Input: part model. Units: mm. Frame: model coordinates. Face numbers are marked on the shaded views. A direction names the side the tool comes from. Give positions to 0.01 mm unless a question says otherwise; leave off trailing zeros. Order: outer loops, then holes, each group sorted by start corner. A loop starts at its lowest first (then second) coordinate and runs counter-clockwise, first axis right, second up. Notation, with made-up numbers: (13, -4) - (17, -4) arc R28 ccw to (17, 18) - close; hole circle Ø10 at (88.25, -2.5). An arc over 180 degrees is marked (long way). Answer in a Markdown table with one row per item. Add a question column.
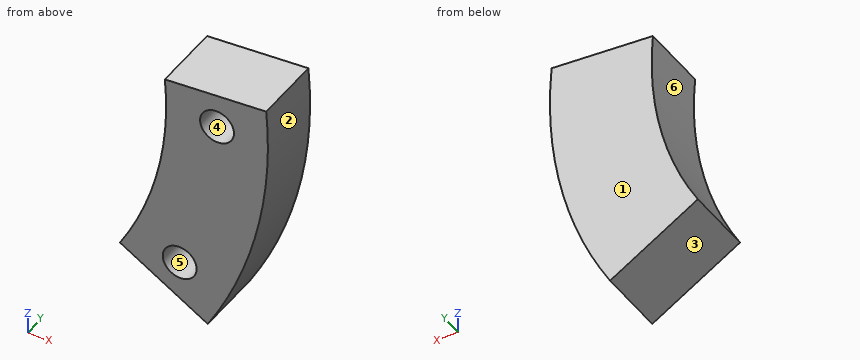
from build123d import *

# Parameters (mm, degrees)
BOSS_EXTRUDE1_DEPTH       = 10
F_5_0MM_DOWEL_HOLE1_D     = 5
F_5_0MM_DOWEL_HOLE1_DEPTH = 6
F_5_0MM_DOWEL_HOLE1_TIP   = 1.502151548


with BuildPart() as part:
    # Sketch1 → Boss-Extrude1 (new body)
    with BuildSketch(Plane(origin=(0, 0, 0), x_dir=(1, 0, 0), z_dir=(0, 1, 0))):
        with BuildLine():
            ThreePointArc((49.589984709, -4.345321229), (48.569954781, 10.909073863), (42.968659609, 25.134492066))
            Line((42.968659609, 25.134492066), (55.916226787, 32.708163842))
            ThreePointArc((55.916226787, 32.708163842), (63.205336897, 14.196259639), (64.532728193, -5.654678771))
            Line((64.532728193, -5.654678771), (49.589984709, -4.345321229))
        make_face()
    extrude(amount=BOSS_EXTRUDE1_DEPTH)

    # Ø5.0mm Dowel Hole1
    with Locations(Plane(origin=(0, 0, 0), x_dir=(-1, 0, 0), z_dir=(0, -1, 0))):
        with Locations((-57.28, 0), (-51.776228177, 24.499399905)):
            Hole(F_5_0MM_DOWEL_HOLE1_D / 2, depth=F_5_0MM_DOWEL_HOLE1_DEPTH)
            with Locations((0, 0, -(F_5_0MM_DOWEL_HOLE1_DEPTH + F_5_0MM_DOWEL_HOLE1_TIP / 2))):  # 118° drill point
                Cone(0, F_5_0MM_DOWEL_HOLE1_D / 2, F_5_0MM_DOWEL_HOLE1_TIP, mode=Mode.SUBTRACT)


solid = part.part
Q1. Section B-B, the plane z = -21. Return loops of the section in (x, y).
Q2. Section A-A, the plane y = 7. Return loops of the section in (x, z), then the cut area to 3 significant figures.
Q3. Contact query for flat-ended pins moving along their axis: P1, Ø1.5, axis at y = 7, z = -21, coming from the +X side; P2, Ø1, axis at y = 7, z = -0.5, coming from the -X side; P3, Ø2, axis at x = 49.5, y = 5.5, coming from the -Z side. Output: stop coordinate, or through.
Q4. Line query: probe 1 along Z at (x, y) = (59.5, 5.75); probe 2 along Z at (x, y) = (55.5, 5); probe 3 along X at (y, z) = (5, -22.5). Output: solid intervals per line, ascending.
Q5. Pull-direction query (Z, two-part tool) for the marked faces 1, 2, 3 and 4; classes: +Z half, -Z half, draft (parallel to the pull), parting line (faces both ways), or undercut.
Q6. Access query for the marked faces 5 and 6. Directions: +Z, -Z, +X, -X, +Y, -Y. A direction counts if a zero-diameter tool reaches every point of the face in a straight line with its end or side. Return the directions, or none.
Q7. Section C-C, the plane z = -28. Return loops of the section in (x, y).
Computed:
| question | item | result |
|---|---|---|
| 1 | outline | (45.13, 0) - (61.28, 0) - (61.28, 10) - (45.13, 10) - close |
| 2 | outline | (42.97, -25.13) - (55.92, -32.71) arc R64.78 ccw to (64.53, 5.65) - (49.59, 4.35) arc R49.78 cw to start; hole circle Ø1.67 at (51.78, -24.5); hole circle Ø1.67 at (57.28, 0) |
| 2 | area | 525 mm^2 |
| 3 | P1 | stops at x = 61.53 |
| 3 | P2 | stops at x = 49.77 |
| 3 | P3 | stops at z = -29.54 |
| 4 | probe 1 | z = -25.62 to -1.15, 1.15 to 5.21 |
| 4 | probe 2 | z = -32.46 to -1.76, 1.76 to 4.86 |
| 4 | probe 3 | x = 44.4 to 50.28, 53.28 to 60.75 |
| 5 | face 1 | draft |
| 5 | face 2 | parting line |
| 5 | face 3 | -Z half |
| 5 | face 4 | undercut |
| 6 | face 5 | -Y |
| 6 | face 6 | -X, +Y, -Y |
| 7 | outline | (47.87, 0) - (58.42, 0) - (58.42, 10) - (47.87, 10) - close |
